The model under review builds one solid part; all positions refer to its coordinate system, in mm. A direction names the side the tool comes from. Coordinates: 2 decimals unless noted, no trailing zeros. Write each loop counter-clockwise with the first axis right and the second up, starting at its lowest first coordinate (ties: lowest second). Pieces come first, ordered by that corner, then holes. Notation, with made-up numbers: (-37.75, 47) - (-12.75, 47) arc R14 cw to (-12.75, 74) - close; hole circle Ø10 at (-20, 80.25). An arc over 180 degrees is marked (long way). Put each result on its own line as item: value.
from build123d import *

# Parameters (mm, degrees)
SKETCH1_R                  = 4.7752
BOSS_EXTRUDE1_DEPTH        = 6.35
F_4_40_TAPPED_HOLE1_REACH  = 112.943
F_4_40_TAPPED_HOLE1_BORE_R = 1.1303


with BuildPart() as part:
    # Sketch1 → Boss-Extrude1 (new body)
    with BuildSketch(Plane(origin=(0, 0, 0), x_dir=(0, 0, -1), z_dir=(1, 0, 0))):
        with BuildLine():
            ThreePointArc((0, -12.7), (12.7, 0), (0, 12.7))
            Line((0, 12.7), (-1.581322957, 12.601167315))
            Line((-1.581322957, 12.601167315), (-101.6, 6.35))
            ThreePointArc((-101.6, 6.35), (-107.95, 0), (-101.6, -6.35))
            Line((-101.6, -6.35), (-1.581322957, -12.601167315))
            Line((-1.581322957, -12.601167315), (0, -12.7))
        make_face()
        with BuildLine():
            Line((-12.7, 6.02134877), (-12.7, -6.02134877))
            ThreePointArc((-12.7, -6.02134877), (-13.500867997, -7.872569955), (-15.398440847, -8.556402319))
            Line((-15.398440847, -8.556402319), (-92.868440847, -3.714527319))
            ThreePointArc((-92.868440847, -3.714527319), (-94.561221185, -2.918605773), (-95.25, -1.17947377))
            Line((-95.25, -1.17947377), (-95.25, 1.17947377))
            ThreePointArc((-95.25, 1.17947377), (-94.561221185, 2.918605773), (-92.868440847, 3.714527319))
            Line((-92.868440847, 3.714527319), (-15.398440847, 8.556402319))
            ThreePointArc((-15.398440847, 8.556402319), (-13.500867997, 7.872569955), (-12.7, 6.02134877))
        make_face(mode=Mode.SUBTRACT)
        Circle(SKETCH1_R, mode=Mode.SUBTRACT)
    extrude(amount=BOSS_EXTRUDE1_DEPTH)

    # #4-40 Tapped Hole1 bore (on position points) → #4-40 Tapped Hole1 (cut, up to next)
    with BuildSketch(Plane(origin=(3.175, 12.7, 0), x_dir=(0, -0.062378286155, 0.998052578483), z_dir=(0, 0.998052578483, 0.062378286155)), mode=Mode.PRIVATE) as f_4_40_tapped_hole1_sk1:
        Circle(F_4_40_TAPPED_HOLE1_BORE_R)
    f_4_40_tapped_hole1_tool1 = extrude(f_4_40_tapped_hole1_sk1.sketch, amount=-F_4_40_TAPPED_HOLE1_REACH, mode=Mode.PRIVATE) & part.part
    add(f_4_40_tapped_hole1_tool1.solids().sort_by_distance((3.175, 12.7, 0))[0], mode=Mode.SUBTRACT)


solid = part.part
1. To check wall thickness, follow probe 1 along Y at (x, z) = (5, 0); probe 2 along Z at (x, y) = (3, -2.75); probe 3 along Y at (x, z) = (3, 0). State the ranges of each line that lie inside material, in increasing order.
Determined:
probe 1: y = -12.7 to -4.78, 4.78 to 12.7
probe 2: z = -12.4 to -3.9, 3.9 to 12.7, 94.71 to 107.32
probe 3: y = -12.7 to -4.78
2. Consider section B-B on z = 48.5. State the section outline as (x, y) points, plus the area to 3 significant figures.
Determined:
outline: (0, -9.67) - (6.35, -9.67) - (6.35, -6.49) - (0, -6.49) - close; (0, 6.49) - (6.35, 6.49) - (6.35, 9.67) - (0, 9.67) - close
area: 40.4 mm^2
3. Consider section C-C on y = -10.75. State the section outline as (x, z) points.
Determined:
outline: (0, -6.76) - (6.35, -6.76) - (6.35, 31.2) - (0, 31.2) - close
4. The part is to be moulded in two halves that separate along Y. For faces 1 (the cylindrical face through (3.13, 0.14, 107.95)), 2 (the flat face through (3.13, -6.17, 53.59)), 3 (the flat face through (0, -8, 35)), say which applies: +Y half, -Y half, draft (parallel to the pull), parting line (faces both ways), or undercut.
Determined:
face 1: parting line
face 2: undercut
face 3: draft
5. For pin 1 Ø1 at (x, z) = (4.5, 13) entering from -Y; pin 2 Ø10 at (y, z) = (5, 65) entering from -X; pin 3 Ø2 at (x, z) = (3.5, 52) entering from +Y; pin 4 Ø1.5 at (x, y) = (5, -5.5) entering from -Z, all flat-tipped, find the tip position at first contact; note any pin that passes through.
Determined:
pin 1: stops at y = -11.92
pin 2: stops at x = 0
pin 3: stops at y = 9.51
pin 4: stops at z = -11.78
6. Machinability: for faces 4 (the flat face through (3, 0, 95.25)), 5 (the cylindrical face through (4.13, 8.57, 0.35)), which of the approach directions +Z, -Z, +X, -X, +Y, -Y give a long, thin tool a straight path to every point of the face, cutting with its end or side? Answer none if there is none.
Determined:
face 4: +X, -X
face 5: none
7. Consider section A-A on y = 0. State the section outline as (x, z) points, plus the area to 3 significant figures.
Determined:
outline: (0, -12.7) - (6.35, -12.7) - (6.35, -4.78) - (0, -4.78) - close; (0, 4.78) - (6.35, 4.78) - (6.35, 12.7) - (0, 12.7) - close; (0, 95.25) - (6.35, 95.25) - (6.35, 107.95) - (0, 107.95) - close
area: 181 mm^2
